```python
from build123d import *

# Parameters (mm, degrees)
SKETCH_1_R      = 1.45
EXTRUDE_1_DEPTH = 2
FILLET_1_R      = 3


with BuildPart() as part:
    # 草图1 → 凸台-拉伸1 (new body)
    with BuildSketch(Plane(origin=(0, 0, 0), x_dir=(1, 0, 0), z_dir=(0, 1, 0))):
        Polygon((0, 15), (0, 0), (30, -20), (45, -20), (60, 0), (60, 15), (52.613356649, 15), (45, 15), (32, 15), (15, 35), (0, 35), align=None)
        Polygon((30, -16.394448725), (5.408326913, 0), (30, 0), align=None, mode=Mode.SUBTRACT)
        with Locations(Location((37.5, -15, 0), (0, 0, 270))):
            Circle(SKETCH_1_R, mode=Mode.SUBTRACT)
        Polygon((45, 0), (56.25, 0), (45, -15), align=None, mode=Mode.SUBTRACT)
        with Locations(Location((37.5, -5, 0), (0, 0, 270))):
            Circle(SKETCH_1_R, mode=Mode.SUBTRACT)
        with Locations(Location((10, 7.5, 0), (0, 0, 270))):
            Circle(SKETCH_1_R, mode=Mode.SUBTRACT)
        with Locations(Location((7.5, 20, 0), (0, 0, 270))):
            Circle(SKETCH_1_R, mode=Mode.SUBTRACT)
        with Locations(Location((7.5, 30, 0), (0, 0, 270))):
            Circle(SKETCH_1_R, mode=Mode.SUBTRACT)
        Polygon((15, 28.82380953), (26.750238101, 15), (15, 15), align=None, mode=Mode.SUBTRACT)
        with Locations(Location((30, 7.5, 0), (0, 0, 270))):
            Circle(SKETCH_1_R, mode=Mode.SUBTRACT)
        with Locations(Location((50, 7.5, 0), (0, 0, 270))):
            Circle(SKETCH_1_R, mode=Mode.SUBTRACT)
    extrude(amount=EXTRUDE_1_DEPTH)

    # 圆角1
    fillet_1_edges = [part.edges().sort_by_distance(p)[0] for p in [
        (15, 1, -15),
        (26.750238101, 1, -15),
        (15, 1, -28.82380953),
        (45, 1, 15),
        (56.25, 1, 0),
        (45, 1, 0),
        (30, 1, 0),
        (5.408326913, 1, 0),
        (30, 1, 16.394448725),
        (60, 1, -15),
        (60, 1, 0),
        (45, 1, 20),
        (30, 1, 20),
        (0, 1, 0),
        (0, 1, -35),
        (15, 1, -35),
        (32, 1, -15),
    ]]
    fillet(fillet_1_edges, radius=FILLET_1_R)


solid = part.part
```
Build history of the part. All positions in model axes, mm. A direction names the side the tool comes from. Coordinates: 2 decimals unless noted, no trailing zeros. Write each loop counter-clockwise with the first axis right and the second up, starting at its lowest first coordinate (ties: lowest second). Pieces come first, ordered by that corner, then holes.
1. 3-axis set-ups, long thin cutter, end or side, ignore diameter. For faces 5 (the cylindrical face through (0.365, 1.014, -0.172)), 6 (the flat face through (19, 1, -15)): which of +Z, -Z, +X, -X, +Y, -Y reach the whole face in a straight line?
Answer block:
face 5: +Z, -X, +Y, -Y
face 6: +Y, -Y
2. Band-saw the part on A-A, the plane z = 15. Give the cut face in (x, y).
Answer block:
outline: (22.5, 0) - (36.05, 0) - (36.05, 2) - (22.5, 2) - close; (38.95, 0) - (48.75, 0) - (48.75, 2) - (38.95, 2) - close
3. Band-saw the part on C-C, the plane z = -7.5. Give the cut face in (x, y), and give its area (3 significant figures).
Answer block:
outline: (0, 0) - (8.55, 0) - (8.55, 2) - (0, 2) - close; (11.45, 0) - (28.55, 0) - (28.55, 2) - (11.45, 2) - close; (31.45, 0) - (48.55, 0) - (48.55, 2) - (31.45, 2) - close; (51.45, 0) - (60, 0) - (60, 2) - (51.45, 2) - close
area: 103 mm2
4. Pull direction Z, two halves, no side cores. Call faces 1 (the cylindrical face through (22.965, 1.014, -16.698)), 2 (the cylindrical face through (30.03, 1.01, 19.87)), 3 (the flat face through (21, 1, 0)), 4 (the cylindrical face through (59.14, 1.01, -14.1)): released by +Z, released by -Z, zero draft, split by the parting line, or undercut.
Answer block:
face 1: undercut
face 2: released by +Z
face 3: undercut
face 4: released by -Z
5. Drop a flat-ended pin along its axis: pin 1 (0.6 mm diameter, centred on x = 50, y = 1.5, fed in from -Z). Give the stop position or say it passes through.
Answer block:
pin 1: stops at z = -15
6. Band-saw the part on B-B, the plane x = 7.5. Give the cut face in (y, z).
Answer block:
outline: (0, -35) - (2, -35) - (2, -31.45) - (0, -31.45) - close; (0, -28.55) - (2, -28.55) - (2, -21.45) - (0, -21.45) - close; (0, -18.55) - (2, -18.55) - (2, 5) - (0, 5) - close
7. Band-saw the part on D-D, the plane y = 0.7. Give the number of separate pieces and of enclosed holes in the cut face, and give its area (3 significant figures).
Answer block:
separate pieces: 1
enclosed holes: 10
area: 1,780 mm2
8. Drill centre lines: probe 1 along X at (y, z) = (1.1, -7.5); probe 2 along X at (y, z) = (1.2, 5); probe 3 along X at (y, z) = (1.05, -20). Where is each one in solid material? Low to high.
Answer block:
probe 1: x = 0 to 8.55, 11.45 to 28.55, 31.45 to 48.55, 51.45 to 60
probe 2: x = 7.5 to 13.08, 30 to 36.05, 38.95 to 45, 52.5 to 56.25
probe 3: x = 0 to 6.05, 8.95 to 15, 22.5 to 27.75
